Could you check a few things on this model? Use its own coordinates, in mm. Face numbers are marked on the shaded views. Give positions to 0.01 mm unless a question says otherwise; leave off trailing zeros. Write each loop counter-clockwise with the first axis right and the second up, starting at its lowest first coordinate (ties: lowest second). Pieces come first, ordered by that corner, then holes. Notation, with made-up numbers: (39.5, 87) - (76.5, 87) arc R14 cw to (76.5, 107) - close; hole circle Ø6 at (83.5, 70.5). An arc over 180 degrees is marked (long way). Use one line per item in the form item = value.
```python
from build123d import *

# Parameters (mm, degrees)
EXTRUDE_1_DEPTH     = 10
EXTRUDE_2_DEPTH     = 10
EXTRUDE_4_DEPTH     = 10
SKETCH_3_R          = 2.25
CUT_EXTRUDE_4_DEPTH = 12.6
SKETCH_4_R          = 2.25
CUT_EXTRUDE_2_DEPTH = 7
FILLET_2_R          = 1
EXTRUDE_3_DEPTH     = 10
CUT_EXTRUDE_3_DEPTH = 11
FILLET_3_R          = 1
FILLET_4_R          = 2


with BuildPart() as part:
    # Эскиз1 → Бобышка-Вытянуть1 (new body)
    with BuildSketch(Plane(origin=(0, 0, 0), x_dir=(1, 0, 0), z_dir=(0, 1, 0))):
        with BuildLine():
            Line((0, 0), (0, 8))
            ThreePointArc((0, 8), (-7.1, 15.1), (0, 22.2))
            Line((0, 22.2), (0, 37.8))
            ThreePointArc((0, 37.8), (-7.1, 44.9), (0, 52))
            Line((0, 52), (0, 60))
            Line((0, 60), (-3, 60))
            Line((-3, 60), (-3, 54.544169223))
            ThreePointArc((-3, 54.544169223), (-10.1, 44.9), (-3, 35.255830777))
            Line((-3, 35.255830777), (-3, 24.744169223))
            ThreePointArc((-3, 24.744169223), (-10.1, 15.1), (-3, 5.455830777))
            Line((-3, 5.455830777), (-3, 0))
            Line((-3, 0), (0, 0))
        make_face()
    extrude(amount=EXTRUDE_1_DEPTH)

    # Эскиз2 → Бобышка-Вытянуть2 (add)
    with BuildSketch(Plane(origin=(0, 10, 0), x_dir=(1, 0, 0), z_dir=(0, 1, 0))):
        with BuildLine():
            Line((-3, 60), (-8.049844719, 60))
            Line((-8.049844719, 60), (-8.049844719, 51))
            ThreePointArc((-8.049844719, 51), (-5.802159163, 53.167100402), (-3, 54.544169223))
            Line((-3, 54.544169223), (-3, 60))
        make_face()
        with BuildLine():
            Line((-3, 0), (-3, 5.455830777))
            ThreePointArc((-3, 5.455830777), (-5.802159163, 6.832899598), (-8.049844719, 9))
            Line((-8.049844719, 9), (-8.049844719, 0))
            Line((-8.049844719, 0), (-3, 0))
        make_face()
    extrude(amount=-EXTRUDE_2_DEPTH)

    # Эскиз9 → Бобышка-Вытянуть4 (add, through all)
    with BuildSketch(Plane.XZ):
        with BuildLine():
            Line((-6, -25.027738917), (-6, -34.972261083))
            ThreePointArc((-6, -34.972261083), (-11.340897297, -42.461958059), (-9.549844719, -51.484866426))
            Line((-9.549844719, -51.484866426), (-9.549844719, -60))
            Line((-9.549844719, -60), (-8.049844719, -60))
            Line((-8.049844719, -60), (-8.049844719, -51))
            ThreePointArc((-8.049844719, -51), (-9.617405222, -41.81527687), (-3, -35.255830777))
            Line((-3, -35.255830777), (-3, -24.744169223))
            ThreePointArc((-3, -24.744169223), (-9.617405222, -18.18472313), (-8.049844719, -9))
            Line((-8.049844719, -9), (-8.049844719, 0))
            Line((-8.049844719, 0), (-9.549844719, 0))
            Line((-9.549844719, 0), (-9.549844719, -8.515133574))
            ThreePointArc((-9.549844719, -8.515133574), (-11.340897297, -17.538041941), (-6, -25.027738917))
        make_face()
    extrude(amount=-EXTRUDE_4_DEPTH)

    # Эскиз3 → Вырез-Вытянуть4 (cut, through all)
    with BuildSketch(Plane.ZY):
        with Locations((-55.75, 5)):
            Circle(SKETCH_3_R)
        with Locations((-4.25, 5)):
            Circle(SKETCH_3_R)
    extrude(amount=CUT_EXTRUDE_4_DEPTH, mode=Mode.SUBTRACT)

    # Эскиз4 → Вырез-Вытянуть2 (cut, through all)
    with BuildSketch(Plane.ZY.offset(6)):
        with Locations((-30, 5)):
            Circle(SKETCH_4_R)
    extrude(amount=-CUT_EXTRUDE_2_DEPTH, mode=Mode.SUBTRACT)

    # Скругление2
    fillet_2_edges = [part.edges().sort_by_distance(p)[0] for p in [
        (0, 5, -60),
        (0, 5, 0),
    ]]
    fillet(fillet_2_edges, radius=FILLET_2_R)

    # Эскиз5 → Бобышка-Вытянуть3 (add, through all)
    with BuildSketch(Plane.XZ):
        with BuildLine():
            Line((0, -8), (0, -8.1))
            ThreePointArc((0, -8.1), (-7, -15.1), (0, -22.1))
            Line((0, -22.1), (0, -22.2))
            ThreePointArc((0, -22.2), (-7.1, -15.1), (0, -8))
        make_face()
        with BuildLine():
            Line((0, -51.9), (0, -52))
            ThreePointArc((0, -52), (-7.1, -44.9), (0, -37.8))
            Line((0, -37.8), (0, -37.9))
            ThreePointArc((0, -37.9), (-7, -44.9), (0, -51.9))
        make_face()
    extrude(amount=-EXTRUDE_3_DEPTH)

    # Эскиз7 → Вырез-Вытянуть3 (cut, through all)
    with BuildSketch(Plane(origin=(0, 10, 0), x_dir=(1, 0, 0), z_dir=(0, 1, 0))):
        with BuildLine():
            Line((0, 51.9), (0, 53.4))
            ThreePointArc((0, 53.4), (-8.5, 44.9), (0, 36.4))
            Line((0, 36.4), (0, 37.9))
            ThreePointArc((0, 37.9), (-7, 44.9), (0, 51.9))
        make_face()
        with BuildLine():
            Line((0, 22.1), (0, 23.6))
            ThreePointArc((0, 23.6), (-8.5, 15.1), (0, 6.6))
            Line((0, 6.6), (0, 8.1))
            ThreePointArc((0, 8.1), (-7, 15.1), (0, 22.1))
        make_face()
    extrude(amount=-CUT_EXTRUDE_3_DEPTH, mode=Mode.SUBTRACT)

    # Скругление3
    fillet_3_edges = [part.edges().sort_by_distance(p)[0] for p in [
        (-9.549844719, 5, 0),
        (-9.549844719, 5, -60),
    ]]
    fillet(fillet_3_edges, radius=FILLET_3_R)

    # Скругление4
    fillet_4_edges = [part.edges().sort_by_distance(p)[0] for p in [
        (-9.549844719, 5, -8.515133574),
        (-9.549844719, 5, -51.484866426),
        (-6, 5, -34.972261083),
        (-6, 5, -25.027738917),
    ]]
    fillet(fillet_4_edges, radius=FILLET_4_R)


solid = part.part
```
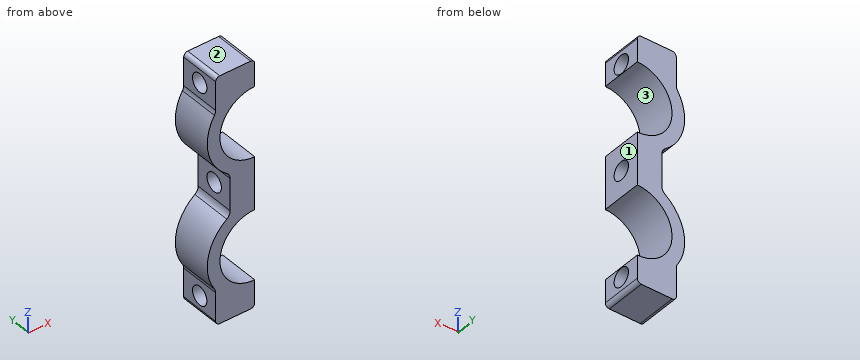
1. Imagine slicing it at D-D, the plane x = -4.5. List the corners of the cut face in (y, z) for me.
Response values:
outline = (0, -60) - (10, -60) - (10, -52.11) - (0, -52.11) - close; (0, -37.69) - (10, -37.69) - (10, -22.31) - (0, -22.31) - close; (0, -7.89) - (10, -7.89) - (10, 0) - (0, 0) - close; hole circle Ø4.5 at (5, -55.75); hole circle Ø4.5 at (5, -30); hole circle Ø4.5 at (5, -4.25)
2. Imagine slicing it at B-B, the plane z = -4.25. List the corners of the cut face in (x, y) for me.
Response values:
outline = (-9.55, 0) - (0, 0) - (0, 2.75) - (-9.55, 2.75) - close; (-9.55, 7.25) - (0, 7.25) - (0, 10) - (-9.55, 10) - close
3. If I drill on line 1 (Z direction, x = -7, y = 6.5); line 2 (Y direction, x = -3.2, z = -30); line 3 (Z direction, x = -6.25, y = 5), over which ranges is the centre line in solid material (lowest first)? Write a range as from..to.
Response values:
line_1 = -60..-57.43, -54.07..-49.72, -40.08..-35.65, -24.35..-19.92, -10.28..-5.93, -2.57..0
line_2 = 0..2.75, 7.25..10
line_3 = -60..-58, -53.5..-50.66, -39.14..-34.87, -25.13..-20.86, -9.34..-6.5, -2..0
4. Imagine slicing it at C-C, the plane x = -7.5. List the corners of the cut face in (y, z) for me, and give its area (3 significant figures).
Response values:
outline = (0, -60) - (10, -60) - (10, -48.9) - (0, -48.9) - close; (0, -40.9) - (10, -40.9) - (10, -36.05) - (0, -36.05) - close; (0, -23.95) - (10, -23.95) - (10, -19.1) - (0, -19.1) - close; (0, -11.1) - (10, -11.1) - (10, 0) - (0, 0) - close; hole circle Ø4.5 at (5, -55.75); hole circle Ø4.5 at (5, -4.25)
area = 287 mm²
5. If we mould it in two halves opening along Z, with no side actions, what happens to the marked faces 1, 2 and 3? For each: pulls with the +Z half, pulls with the -Z half, needs draft (parallel to the pull), parting line crosses it, or undercut.
Response values:
face_1 = needs draft
face_2 = pulls with the +Z half
face_3 = undercut
6. Imagine slicing it at A-A, the plane y = 5. State how many separate pieces and enclosed holes the cut face has, and give its area (3 significant figures).
Response values:
separate_pieces = 4
enclosed_holes = 0
area = 224 mm²
7. For pin 1 (5 mm diameter, centred on y = 6, z = -38.5, fed in from -X); pin 2 (4 mm diameter, centred on y = 5.5, z = -31.5, fed in from -X); pin 3 (1 mm diameter, centred on y = 2, z = -51, fed in from -X), each with a flat end and sliding along its axis, tell me the tip position at first contact or that it passes through.
Response values:
pin_1 = -10.92
pin_2 = -6
pin_3 = -10.16
